Build history of the part. All positions in model axes, mm. Face numbers are marked on the shaded views. Give positions to 0.01 mm unless a question says otherwise; leave off trailing zeros. Order: outer loops, then holes, each group sorted by start corner. A loop starts at its lowest first (then second) coordinate and runs counter-clockwise, first axis right, second up. Notation, with made-up numbers: (44.5, 37.25) - (77.5, 37.25) arc R18 ccw to (77.5, 54.25) - close; hole circle Ø7 at (36, 73). An arc over 180 degrees is marked (long way). Use a Markdown table: item, result. Add a question column.
(1) Flat gauge pins, fed straight in: pin 1 (2.5 mm diameter, centred on y = 33.5, z = 9, fed in from -X) (3 decimals); pin 2 (4 mm diameter, centred on y = 73.5, z = 14, fed in from +X) (3 decimals); pin 3 (1.5 mm diameter, centred on x = 259.5, y = 50, fed in from -Z); pin 4 (10.5 mm diameter, centred on y = 70.5, z = 10, fed in from -X) (3 decimals). Where does each tip first touch, or does it go through?
(2) Slice it at B-B (x = 16). Write the cut outline in (y, z), then the cut area to 3 significant figures.
(3) Wall check: line 1 (Y direction, x = 161, z = 7.75); line 2 (X direction, y = 43, z = 12); line 3 (X direction, y = -6.5, z = 3). Give the ranges that are in metal, low to high.
(4) Slice it at A-A (x = 167). Write the cut outline in (y, z).
(5) Mould opens along X. For the marked faces 1, 2 and 3 say: +X half, -X half, draft (parallel to the pull), parting line (faces both ways), or undercut.
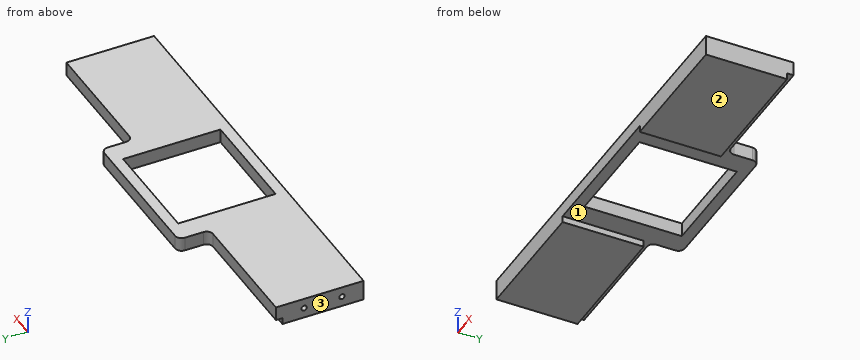
from build123d import *

# Parameters (mm, degrees)
F0_W     = 120
F0_H     = 6
F0_W_2   = 6
F0_H_2   = 23
F0_H_3   = 75
F1_DEPTH = 19
F2_DEPTH = 6
F3_R     = 6
F4_R     = 2.5
F5_DEPTH = 25


with BuildPart() as f1:
    # F0 (on Top) → F1 (new body)
    with BuildSketch(Plane.XY):
        with Locations((29.2149764299, 55.6197040975)):
            Rectangle(F0_W, F0_H)
        with Locations((92.2149764299, 70.1197040975)):
            Rectangle(F0_W_2, F0_H_2)
        with Locations((92.2149764299, 55.6197040975)):
            Rectangle(F0_W_2, F0_H)
        with Locations((29.2149764299, 15.1197040975)):
            Rectangle(F0_W, F0_H_3)
        Polygon((109.2149764299, 58.6197040975), (95.2149764299, 58.6197040975), (95.2149764299, 52.6197040975), (89.2149764299, 52.6197040975), (89.2149764299, -22.3802959025), (159.2149764299, -22.3802959025), (159.2149764299, -12.3802959025), (109.2149764299, -12.3802959025), align=None)
        Polygon((89.2149764299, 87.6197040975), (89.2149764299, 81.6197040975), (95.2149764299, 81.6197040975), (159.2149764299, 81.6197040975), (159.2149764299, 87.6197040975), align=None)
        Polygon((159.2149764299, 87.6197040975), (159.2149764299, 81.6197040975), (223.2149764299, 81.6197040975), (229.2149764299, 81.6197040975), (229.2149764299, 87.6197040975), align=None)
        Polygon((159.2149764299, -12.3802959025), (159.2149764299, -22.3802959025), (229.2149764299, -22.3802959025), (229.2149764299, 52.6197040975), (229.2137485743, 52.6197040975), (223.2149764299, 52.6197040975), (223.2149764299, 58.6197040975), (209.2149764299, 58.6197040975), (209.2149764299, -12.3802959025), align=None)
        with Locations((226.2149764299, 70.1197040975)):
            Rectangle(F0_W_2, F0_H_2)
        with Locations((289.2149764299, 15.1197040975)):
            Rectangle(F0_W, F0_H_3)
        Polygon((229.2149764299, 58.6197040975), (223.2149764299, 58.6197040975), (223.2149764299, 52.6197040975), (229.2137485743, 52.6197040975), (229.2149764299, 52.6197040975), align=None)
        with Locations((289.2149764299, 55.6197040975)):
            Rectangle(F0_W, F0_H)
        Polygon((95.2149764299, 81.6197040975), (95.2149764299, 58.6197040975), (109.2149764299, 58.6197040975), (109.2149764299, 77.6197040975), (159.2149764299, 77.6197040975), (159.2149764299, 81.6197040975), align=None)
        Polygon((223.2149764299, 81.6197040975), (159.2149764299, 81.6197040975), (159.2149764299, 77.6197040975), (209.2149764299, 77.6197040975), (209.2149764299, 58.6197040975), (223.2149764299, 58.6197040975), align=None)
    extrude(amount=F1_DEPTH)

    # F0 (on Top) → F2 (cut)
    with BuildSketch(Plane.XY):
        with Locations((29.2149764299, 55.6197040975)):
            Rectangle(F0_W, F0_H)
        with Locations((92.2149764299, 55.6197040975)):
            Rectangle(F0_W_2, F0_H)
        with Locations((289.2149764299, 55.6197040975)):
            Rectangle(F0_W, F0_H)
        with Locations((92.2149764299, 70.1197040975)):
            Rectangle(F0_W_2, F0_H_2)
        Polygon((89.2149764299, 87.6197040975), (89.2149764299, 81.6197040975), (95.2149764299, 81.6197040975), (159.2149764299, 81.6197040975), (159.2149764299, 87.6197040975), align=None)
        Polygon((159.2149764299, 87.6197040975), (159.2149764299, 81.6197040975), (223.2149764299, 81.6197040975), (229.2149764299, 81.6197040975), (229.2149764299, 87.6197040975), align=None)
        with Locations((226.2149764299, 70.1197040975)):
            Rectangle(F0_W_2, F0_H_2)
        Polygon((229.2149764299, 58.6197040975), (223.2149764299, 58.6197040975), (223.2149764299, 52.6197040975), (229.2137485743, 52.6197040975), (229.2149764299, 52.6197040975), align=None)
        Polygon((159.2149764299, -12.3802959025), (159.2149764299, -22.3802959025), (229.2149764299, -22.3802959025), (229.2149764299, 52.6197040975), (229.2137485743, 52.6197040975), (223.2149764299, 52.6197040975), (223.2149764299, 58.6197040975), (209.2149764299, 58.6197040975), (209.2149764299, -12.3802959025), align=None)
        Polygon((109.2149764299, 58.6197040975), (95.2149764299, 58.6197040975), (95.2149764299, 52.6197040975), (89.2149764299, 52.6197040975), (89.2149764299, -22.3802959025), (159.2149764299, -22.3802959025), (159.2149764299, -12.3802959025), (109.2149764299, -12.3802959025), align=None)
        Polygon((223.2149764299, 81.6197040975), (159.2149764299, 81.6197040975), (159.2149764299, 77.6197040975), (209.2149764299, 77.6197040975), (209.2149764299, 58.6197040975), (223.2149764299, 58.6197040975), align=None)
        Polygon((95.2149764299, 81.6197040975), (95.2149764299, 58.6197040975), (109.2149764299, 58.6197040975), (109.2149764299, 77.6197040975), (159.2149764299, 77.6197040975), (159.2149764299, 81.6197040975), align=None)
    extrude(amount=F2_DEPTH, mode=Mode.SUBTRACT)

    # F3
    f3_edges = [f1.edges().sort_by_distance(p)[0] for p in [
        (229.214976, 58.619704, 12.5),
        (229.214976, 87.619704, 12.5),
        (89.214976, 87.619704, 12.5),
        (89.214976, 58.619704, 12.5),
    ]]
    fillet(f3_edges, radius=F3_R)

    # F4 (on face) → F5 (cut)
    with BuildSketch(Plane(origin=(-30.7850235701, 0, 0), x_dir=(0, -1, 0), z_dir=(-1, 0, 0))):
        with Locations((-32.6197040975, 9.5)):
            Circle(F4_R)
        with Locations((2.3802959025, 9.5)):
            Circle(F4_R)
    extrude(amount=-F5_DEPTH, mode=Mode.SUBTRACT)


solid = f1.part
Solution:
| question | item | result |
|---|---|---|
| 1 | pin 1 | x = -5.785 |
| 1 | pin 2 | x = 229.215 |
| 1 | pin 3 | z = 0 |
| 1 | pin 4 | x = 89.215 |
| 2 | outline | (-22.38, 0) - (52.62, 0) - (52.62, 6) - (58.62, 6) - (58.62, 19) - (-22.38, 19) - close |
| 2 | area | 1,500 mm2 |
| 3 | line 1 | -22.38 to -12.38, 77.62 to 87.62 |
| 3 | line 2 | -30.79 to 109.21, 209.21 to 349.21 |
| 3 | line 3 | -30.79 to 89.21, 229.21 to 349.21 |
| 4 | outline | (-22.38, 6) - (-12.38, 6) - (-12.38, 19) - (-22.38, 19) - close; (77.62, 6) - (87.62, 6) - (87.62, 19) - (77.62, 19) - close |
| 5 | face 1 | undercut |
| 5 | face 2 | draft |
| 5 | face 3 | -X half |
